```python
from build123d import *

# Parameters (mm, degrees)
SKETCH1_R           = 12.5
BOSS_EXTRUDE1_DEPTH = 10.5
CHAMFER1_SIZE       = 0.1
SKETCH4_R           = 3.51
CUT_EXTRUDE1_DEPTH  = 1
SKETCH5_R           = 3.5
BOSS_EXTRUDE2_DEPTH = 3.5
CUT_EXTRUDE2_REACH  = 31.407
SKETCH6_R           = 2
SKETCH7_R           = 4
CUT_EXTRUDE3_DEPTH  = 5
CHAMFER2_SIZE       = 0.2
CUT_EXTRUDE4_REACH  = 29.45
SKETCH8_R           = 1.25
SKETCH9_R           = 2.5
CUT_EXTRUDE5_DEPTH  = 3
CHAMFER3_SIZE       = 0.25


with BuildPart() as part:
    # Sketch1 → Boss-Extrude1 (new, symmetric)
    with BuildSketch(Plane.XY):
        with Locations(Location((0, 0, 0), (0, 0, 180))):
            Circle(SKETCH1_R)
    extrude(amount=BOSS_EXTRUDE1_DEPTH, both=True)

    # Sketch2 → Cut-Revolve1 (revolve, cut)
    with BuildSketch(Plane(origin=(0, 0, 0), x_dir=(0, 0, -1), z_dir=(1, 0, 0)), mode=Mode.PRIVATE) as cut_revolve1_sk:
        Polygon((-6.15, 12.5), (-6.05, 12.5), (-6.1, 12.45), align=None)
        Polygon((6.05, 12.5), (6.15, 12.5), (6.1, 12.45), align=None)
    revolve(cut_revolve1_sk.sketch.rotate(Axis((0, 0, 10.5), (0, 0, -1)), 270), axis=Axis((0, 0, 10.5), (0, 0, -1)), mode=Mode.SUBTRACT)

    # Chamfer1
    chamfer1_edges = [part.edges().sort_by_distance(p)[0] for p in [
        (12.5, 0, -10.5),
        (12.5, 0, 10.5),
    ]]
    chamfer(chamfer1_edges, length=CHAMFER1_SIZE)

    # Sketch4 → Cut-Extrude1 (cut)
    with BuildSketch(Plane(origin=(0, 0, -10.5), x_dir=(-1, 0, 0), z_dir=(0, 0, -1))):
        Circle(SKETCH4_R)
    extrude(amount=-CUT_EXTRUDE1_DEPTH, mode=Mode.SUBTRACT)

    # Sketch5 → Boss-Extrude2 (add)
    with BuildSketch(Plane(origin=(0, 0, -9.5), x_dir=(-1, 0, 0), z_dir=(0, 0, -1))):
        Circle(SKETCH5_R)
    extrude(amount=BOSS_EXTRUDE2_DEPTH)

    # Sketch6 → Cut-Extrude2 (cut, up to next)
    with BuildSketch(Plane(origin=(0, 0, -13), x_dir=(-1, 0, 0), z_dir=(0, 0, -1)), mode=Mode.PRIVATE) as cut_extrude2_sk1:
        Circle(SKETCH6_R)
    cut_extrude2_tool1 = extrude(cut_extrude2_sk1.sketch, amount=-CUT_EXTRUDE2_REACH, mode=Mode.PRIVATE) & part.part
    add(cut_extrude2_tool1.solids().sort_by_distance((0, 0, -13))[0], mode=Mode.SUBTRACT)

    # Sketch7 → Cut-Extrude3 (cut)
    with BuildSketch(Plane.XY.offset(10.5)):
        Circle(SKETCH7_R)
    extrude(amount=-CUT_EXTRUDE3_DEPTH, mode=Mode.SUBTRACT)

    # Chamfer2
    chamfer2_edges = [part.edges().sort_by_distance(p)[0] for p in [
        (3.5, 0, -13),
        (2, 0, -13),
    ]]
    chamfer(chamfer2_edges, length=CHAMFER2_SIZE)

    # Sketch8 → Cut-Extrude4 (cut, up to next)
    with BuildSketch(Plane(origin=(0, 0, -10.5), x_dir=(-1, 0, 0), z_dir=(0, 0, -1)), mode=Mode.PRIVATE) as cut_extrude4_sk1:
        with Locations((0, 8.5)):
            Circle(SKETCH8_R)
    cut_extrude4_tool1 = extrude(cut_extrude4_sk1.sketch, amount=-CUT_EXTRUDE4_REACH, mode=Mode.PRIVATE) & part.part
    # Sketch8 → Cut-Extrude4 (cut, up to next)
    with BuildSketch(Plane(origin=(0, 0, -10.5), x_dir=(-1, 0, 0), z_dir=(0, 0, -1)), mode=Mode.PRIVATE) as cut_extrude4_sk2:
        with Locations((8.5, 0)):
            Circle(SKETCH8_R)
    cut_extrude4_tool2 = extrude(cut_extrude4_sk2.sketch, amount=-CUT_EXTRUDE4_REACH, mode=Mode.PRIVATE) & part.part
    # Sketch8 → Cut-Extrude4 (cut, up to next)
    with BuildSketch(Plane(origin=(0, 0, -10.5), x_dir=(-1, 0, 0), z_dir=(0, 0, -1)), mode=Mode.PRIVATE) as cut_extrude4_sk3:
        with Locations((0, -8.5)):
            Circle(SKETCH8_R)
    cut_extrude4_tool3 = extrude(cut_extrude4_sk3.sketch, amount=-CUT_EXTRUDE4_REACH, mode=Mode.PRIVATE) & part.part
    # Sketch8 → Cut-Extrude4 (cut, up to next)
    with BuildSketch(Plane(origin=(0, 0, -10.5), x_dir=(-1, 0, 0), z_dir=(0, 0, -1)), mode=Mode.PRIVATE) as cut_extrude4_sk4:
        with Locations((-8.5, 0)):
            Circle(SKETCH8_R)
    cut_extrude4_tool4 = extrude(cut_extrude4_sk4.sketch, amount=-CUT_EXTRUDE4_REACH, mode=Mode.PRIVATE) & part.part
    add(cut_extrude4_tool1.solids().sort_by_distance((0, 8.5, -10.5))[0], mode=Mode.SUBTRACT)
    add(cut_extrude4_tool2.solids().sort_by_distance((-8.5, 0, -10.5))[0], mode=Mode.SUBTRACT)
    add(cut_extrude4_tool3.solids().sort_by_distance((0, -8.5, -10.5))[0], mode=Mode.SUBTRACT)
    add(cut_extrude4_tool4.solids().sort_by_distance((8.5, 0, -10.5))[0], mode=Mode.SUBTRACT)

    # Sketch9 → Cut-Extrude5 (cut)
    with BuildSketch(Plane(origin=(0, 0, -10.5), x_dir=(-1, 0, 0), z_dir=(0, 0, -1))):
        with Locations((-8.5, 0)):
            Circle(SKETCH9_R)
        with Locations((8.5, 0)):
            Circle(SKETCH9_R)
    extrude(amount=-CUT_EXTRUDE5_DEPTH, mode=Mode.SUBTRACT)

    # Chamfer3
    chamfer3_edges = [part.edges().sort_by_distance(p)[0] for p in [
        (11, 0, -10.5),
        (-6, 0, -10.5),
    ]]
    chamfer(chamfer3_edges, length=CHAMFER3_SIZE)


solid = part.part
```
Geometry: final body of the model. Coordinates: model frame, mm. A direction names the side the tool comes from. Coordinates: 2 decimals unless noted, no trailing zeros. Order: outer loops, then holes, each group sorted by start corner. A loop starts at its lowest first (then second) coordinate and runs counter-clockwise, first axis right, second up. Notation, with made-up numbers: (72.25, 64.25) -> (109.25, 64.25) arc R17 cw to (109.25, 89.25) -> close; hole circle Ø8 at (-28, 42). An arc over 180 degrees is marked (long way). Write item = value, one per line.
(1) Pin query (flat end, axial travel): pin 1 Ø8 at (x, y) = (-10, 4.5) entering from -Z; pin 2 Ø12 at (x, z) = (-2.5, -3.5) entering from -Y; pin 3 Ø5 at (x, z) = (5.5, -6.5) entering from +Y; pin 4 Ø1.5 at (y, z) = (9.5, 6.5) entering from -X. Return the tip coordinate at first contact, or that it passes through.
Solved:
pin_1 = -10.5
pin_2 = -12.5
pin_3 = 12.13
pin_4 = -8.93
(2) Line query: line 1 (Y direction, x = 0, z = -4.25); line 2 (X direction, y = -1, z = 3.75); line 3 (Y direction, x = -0.25, z = 8.5). Output: solid intervals per line, ascending.
Solved:
line_1 = -12.5 to -9.75, -7.25 to -2, 2 to 7.25, 9.75 to 12.5
line_2 = -12.46 to -9.25, -7.75 to -1.73, 1.73 to 7.75, 9.25 to 12.46
line_3 = -12.5 to -9.72, -7.28 to -3.99, 3.99 to 7.28, 9.72 to 12.5
(3) Cut plane B-B on y = 0. Count the separate pieces of the cut face and the enclosed holes in it, plus the area to 3 significant figures.
Solved:
separate_pieces = 4
enclosed_holes = 0
area = 308 mm²
(4) Cut plane A-A on z = -8. Return loops of the section in (x, y).
Solved:
outline = circle Ø25 at (0, 0); hole circle Ø5 at (-8.5, 0); hole circle Ø4 at (0, 0); hole circle Ø2.5 at (0, -8.5); hole circle Ø2.5 at (0, 8.5); hole circle Ø5 at (8.5, 0)
(5) Cut plane C-C on z = -0.75. Return loops of the section in (x, y), plus the area to 3 significant figures.
Solved:
outline = circle Ø25 at (0, 0); hole circle Ø2.5 at (-8.5, 0); hole circle Ø4 at (0, 0); hole circle Ø2.5 at (0, -8.5); hole circle Ø2.5 at (0, 8.5); hole circle Ø2.5 at (8.5, 0)
area = 459 mm²
(6) Access query for faces 4 (the cylindrical face through (9.75, 0.05, 1.37)), 5 (the cylindrical face through (11, 0, -9)). Directions: +Z, -Z, +X, -X, +Y, -Y. A direction counts if a zero-diameter tool reaches every point of the face in a straight line with its end or side. Return the directions, or none.
Solved:
face_4 = +Z, -Z
face_5 = -Z
(7) Pull-direction query (Y, two-part tool) for faces 1 (the cylindrical face through (-11.923, -3.755, -8.245)), 2 (the flat face through (-2, -1, 5.5)), 3 (the flat face through (-3, 3, -10.5)); classes: pulls with the +Y half, pulls with the -Y half, needs draft (parallel to the pull), parting line crosses it, or undercut.
Solved:
face_1 = parting line crosses it
face_2 = undercut
face_3 = needs draft
